```python
from build123d import *

# Parameters (mm, degrees)
SCHIZZO1_R                   = 1
ESTRUSIONE_ESTRUSIONE1_DEPTH = 16
SCHIZZO2_R                   = 2.05
ESTRUSIONE_ESTRUSIONE2_DEPTH = 1.2
RACCORDO1_R                  = 0.5
TAGLIO_ESTRUSIONE1_DEPTH     = 0.5


with BuildPart() as part:
    # Schizzo1 → Estrusione-Estrusione1 (new body)
    with BuildSketch(Plane.XY):
        Circle(SCHIZZO1_R)
    extrude(amount=ESTRUSIONE_ESTRUSIONE1_DEPTH)

    # Schizzo2 → Estrusione-Estrusione2 (add)
    with BuildSketch(Plane(origin=(0, 0, 0), x_dir=(-1, 0, 0), z_dir=(0, 0, -1))):
        Circle(SCHIZZO2_R)
    extrude(amount=ESTRUSIONE_ESTRUSIONE2_DEPTH)

    # Raccordo1
    raccordo1_edges = [part.edges().sort_by_distance(p)[0] for p in [
        (2.05, 0, -1.2),
    ]]
    fillet(raccordo1_edges, radius=RACCORDO1_R)

    # Schizzo3 → Taglio-Estrusione1 (cut)
    with BuildSketch(Plane(origin=(0, 0, -1.2), x_dir=(-1, 0, 0), z_dir=(0, 0, -1))):
        Polygon((-0.25, 0.25), (-1, 0.25), (-1, -0.25), (-0.25, -0.25), (-0.25, -1), (0.25, -1), (0.25, -0.25), (1, -0.25), (1, 0.25), (0.25, 0.25), (0.25, 1), (-0.25, 1), align=None)
    extrude(amount=-TAGLIO_ESTRUSIONE1_DEPTH, mode=Mode.SUBTRACT)


solid = part.part
```
Model file for the job. Use its own axes, mm. Coordinates: 2 decimals unless noted, no trailing zeros. Order: outer loops, then holes, each group sorted by start corner. A loop starts at its lowest first (then second) coordinate and runs counter-clockwise, first axis right, second up. Notation, with made-up numbers: (-30, 63.25) -> (-24, 63.25) arc R10 ccw to (-24, 82.25) -> close; hole circle Ø10 at (34.5, -19.75). An arc over 180 degrees is marked (long way). Answer as a JSON object with one key per item and string values. Group by question number.
1) Cut at A-A, the plane y = 0. Write the cut outline in (x, z).
2) Flat gauge pins, fed straight in: pin 1 (1.5 mm diameter, centred on y = -1.5, z = 10.5, fed in from +X); pin 2 (1.5 mm diameter, centred on x = 0, z = 8, fed in from -Y); pin 3 (0.6 mm diameter, centred on x = -0.5, z = -1, fed in from -Y). Where does each tip first touch, or does it go through?
3) Cut at C-C, the plane z = 12.25. Write the cut outline in (x, y), then the cut area to 3 significant figures.
4) Pull direction Y, two halves, no side cores. Call faces 1 (the face through (0, 0, -0.7)), 2 (the face through (0, -1, 8)), 3 (the face through (0.4, 0.4, -1.2)): +Y half, -Y half, draft (parallel to the pull), parting line (faces both ways), or undercut.
5) Drill centre lines: L1, parallel to Z at x = 0.1, y = -0.2; L2, parallel to Z at x = -0.85, y = 0.8; L3, parallel to X at y = 0.05, z = 3. Where is each one in solid material? Low to high.
Check values:
{
 "1": {"outline": "(-2.05, -0.7) arc R0.5 ccw to (-1.55, -1.2) -> (-1, -1.2) -> (-1, -0.7) -> (1, -0.7) -> (1, -1.2) -> (1.55, -1.2) arc R0.5 ccw to (2.05, -0.7) -> (2.05, 0) -> (1, 0) -> (1, 16) -> (-1, 16) -> (-1, 0) -> (-2.05, 0) -> close"},
 "2": {"pin 1": "stops at x = 0.66", "pin 2": "stops at y = -1", "pin 3": "stops at y = -2.02"},
 "3": {"outline": "circle Ø2 at (0, 0)", "area": "3.14 mm²"},
 "4": {"face 1": "undercut", "face 2": "parting line", "face 3": "draft"},
 "5": {"L1": "z = -0.7 to 16", "L2": "z = -1.2 to 0", "L3": "x = -1 to 1"}
}
